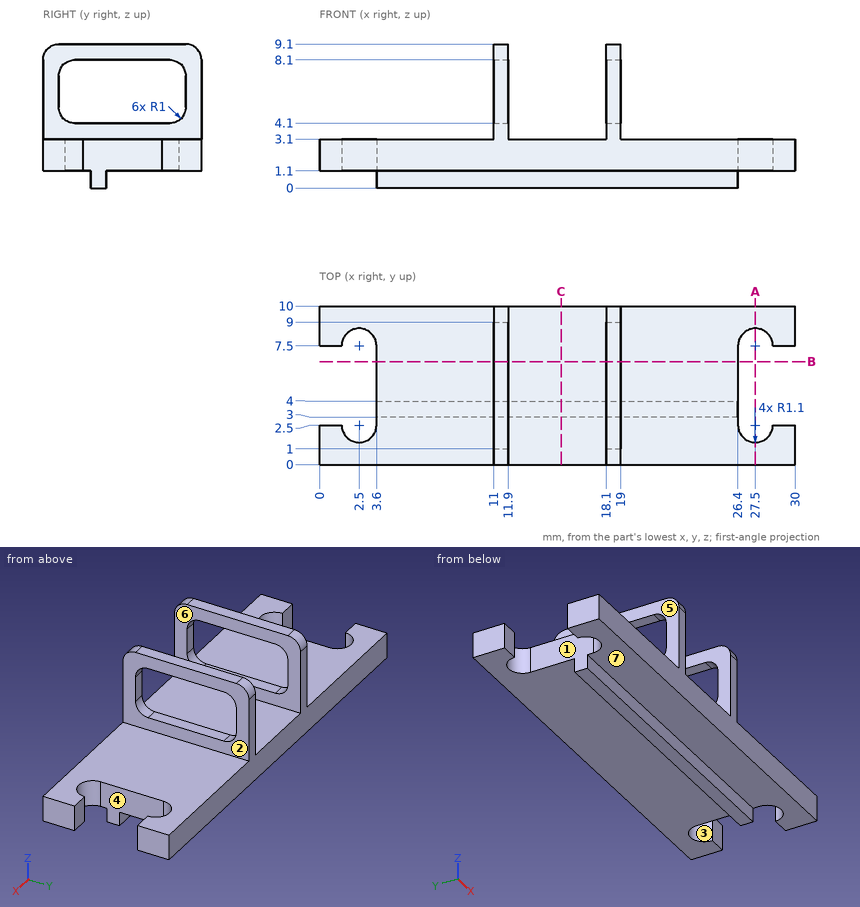
Design review of the part shown in the three views and the two pictorial views. Dimensions are in mm from the part's minimum x, y and z. A direction names the side the tool comes from. Round coordinates to 2 decimals unless told otherwise and drop trailing zeros. Write each loop counter-clockwise with the first axis right and the second up, starting at its lowest first coordinate (ties: lowest second). Pieces come first, ordered by that corner, then holes.
Item 1: We need section B-B on y = 6.5. Write out the cut boundary in (x, z), and give its area (3 significant figures).
Item 2: The part is to be moulded in two halves that separate along X. For the marked faces 5, 6 and 7, say which applies: +X half, -X half, draft (parallel to the pull), parting line (faces both ways), or undercut.
Item 3: We need section C-C on x = 15.25. Write out the cut boundary in (y, z), and give its area (3 significant figures).
Item 4: For the marked faces 1, 2, 3 and 4, list the 3-axis set-ups (+Z, -Z, +X, -X, +Y, -Y) from which the entire face can be reached by the end or side of a thin tool; tool diameter is ignored.
Item 5: For probe 1 along X at (y, z) = (6.25, 3.75); probe 2 along Z at (x, y) = (11.75, 5.25); probe 3 along X at (y, z) = (8, 2), list the stretches that pass through material, from the lowest coordinate up.
Item 6: We need section A-A on x = 27.5. Write out the cut boundary in (y, z).
Item 7: Clearance check with flat-ended pins moving along their axes: pin 1 Ø1.5 at (x, y) = (23.5, 2) entering from -Z; pin 2 Ø0.6 at (x, z) = (14.5, 0.5) entering from +Y; pin 3 Ø3 at (y, z) = (6.5, 6.5) entering from +X; pin 4 Ø3 at (x, y) = (5.5, 2.5) entering from +Z. State where each tip first meets the part, or that it passes through.
Returned:
1. outline: (3.6, 1.1) - (26.4, 1.1) - (26.4, 3.1) - (19, 3.1) - (19, 4.1) - (18.1, 4.1) - (18.1, 3.1) - (11.9, 3.1) - (11.9, 4.1) - (11, 4.1) - (11, 3.1) - (3.6, 3.1) - close; (11, 8.1) - (11.9, 8.1) - (11.9, 9.1) - (11, 9.1) - close; (18.1, 8.1) - (19, 8.1) - (19, 9.1) - (18.1, 9.1) - close
1. area: 49.2 mm2
2. face 5: -X half
2. face 6: undercut
2. face 7: draft
3. outline: (0, 1.1) - (3, 1.1) - (3, 0) - (4, 0) - (4, 1.1) - (10, 1.1) - (10, 3.1) - (0, 3.1) - close
3. area: 21.1 mm2
4. face 1: +Z, -Z, -X
4. face 2: +Z, +X, +Y, -Y
4. face 3: +Z, -Z
4. face 4: +Z, -Z, +X
5. probe 1: x = 11 to 11.9, 18.1 to 19
5. probe 2: z = 1.1 to 4.1, 8.1 to 9.1
5. probe 3: x = 0 to 1.52, 3.48 to 26.52, 28.48 to 30
6. outline: (0, 1.1) - (1.4, 1.1) - (1.4, 3.1) - (0, 3.1) - close; (8.6, 1.1) - (10, 1.1) - (10, 3.1) - (8.6, 3.1) - close
7. pin 1: stops at z = 1.1
7. pin 2: stops at y = 4
7. pin 3: passes through
7. pin 4: stops at z = 3.1
